Here's how the part is built. I have some questions about the finished solid (model axes, mm). Face numbers are marked on the shaded views. A direction names the side the tool comes from. Round coordinates to 2 decimals unless told otherwise and drop trailing zeros. Write each loop counter-clockwise with the first axis right and the second up, starting at its lowest first coordinate (ties: lowest second). Pieces come first, ordered by that corner, then holes. Notation, with made-up numbers: (55.5, -40) -> (100.5, -40) arc R25 cw to (100.5, -1) -> close; hole circle Ø5 at (-11.75, 45). An arc over 180 degrees is marked (long way). Put each result on its own line as item: value. Start each with the question number.
1) I want a section at C-C, the plane z = 10.25. List the corners of the cut face in (x, y) for me (3 decimals).
2) I want a section at D-D, the plane z = 4.75. List the corners of the cut face in (x, y) for me.
3) We'd pull the mould along X, two halves only. Please class the marked faces 3, 4, 5 and 6: released by +X, released by -X, zero draft, split by the parting line, or undercut.
4) If I drill on line 1 along Y through (x, z) = (0.25, 4.75); line 2 along Y through (x, z) = (0, 12.2) (3 decimals); line 3 along Z through (x, y) = (9.5, 2), over which ranges is the centre line in solid material (lowest first)? Write a range as [from, to].
5) Which directions (+Z, -Z, +X, -X, +Y, -Y) give clear straight access to the entire face, cutting with the end or side of a thin tool? Please do the marked faces 1 and 2.
6) Will these pins go through, and if not, where does the flat tip stop? P1, Ø1.5, axis at x = 1.5, z = 6.5, coming from the +Y side; P2, Ø10.5, axis at x = -1.5, y = 1, coming from the +Z side; P3, Ø3, axis at x = 7, z = 5.5, coming from the -Y side; P4, Ø1.5, axis at y = -5.5, z = 7, coming from the +X side.
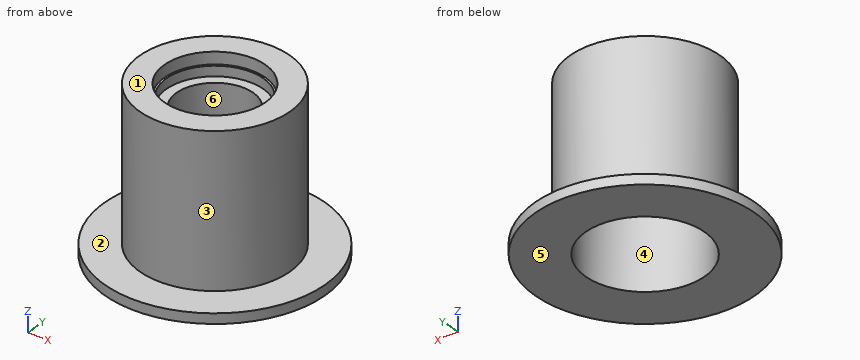
from build123d import *

# Parameters (mm, degrees)
F0_R         = 11
F1_DEPTH     = 1
F2_R         = 7.5
F3_DEPTH     = 15
F4_R         = 3.825
F5_DEPTH     = 25
F6_R         = 5.95
F7_DEPTH     = 7.3
F8_R         = 5.0375
F8_R_2       = 3.825
F9_DEPTH     = 1.2
F10_S5_R     = 5.95
F10_T6_DEPTH = 10
F11_R        = 4.834999796
F11_R_2      = 3.825
F12_DEPTH    = 1


# Not quite as in the source:
# - a fillet or chamfer that OpenCascade refuses, or shapes differently, is made with other operations: its cross-section is extruded or revolved along the edge and cut away or added


with BuildPart() as f1:
    # F0 (on Top) → F1 (new body)
    with BuildSketch(Plane.XY):
        Circle(F0_R)
    extrude(amount=F1_DEPTH)

    # F2 (on face) → F3 (join)
    with BuildSketch(Plane.XY.offset(1)):
        Circle(F2_R)
    extrude(amount=F3_DEPTH)

    # F4 (on face) → F5 (cut)
    with BuildSketch(Plane.XY.offset(16)):
        Circle(F4_R)
    extrude(amount=-F5_DEPTH, mode=Mode.SUBTRACT)

    # F6 (on face) → F7 (cut)
    with BuildSketch(Plane(origin=(0, 0, 0), x_dir=(1, 0, 0), z_dir=(0, 0, -1))):
        Circle(F6_R)
    extrude(amount=-F7_DEPTH, mode=Mode.SUBTRACT)

    # F8 (on face) → F9 (cut)
    with BuildSketch(Plane.XY.offset(16)):
        Circle(F8_R)
        Circle(F8_R_2, mode=Mode.SUBTRACT)
    extrude(amount=-F9_DEPTH, mode=Mode.SUBTRACT)

    # F10: chamfer of 2.2 x 2 on 1 edges, made by hand


with BuildPart() as f10_tool2:
    # F10_s3 → F10_t4 (revolve)
    with BuildSketch(Plane.XZ):
        Polygon((6.025, 7.3), (3.825, 9.3), (3.825, 7.3), align=None)
    revolve(axis=Axis((0, 0, 7.3), (0, 0, 1)))

    # F10_s5 → F10_t6 (intersect, symmetric)
    with BuildSketch(Plane.XY.offset(8.3)):
        Circle(F10_S5_R)
    extrude(amount=F10_T6_DEPTH, both=True, mode=Mode.INTERSECT)


with BuildPart() as f1_1:
    add(f1.part)

    # F10_t1: cut F10_tool2
    add(f10_tool2.part, mode=Mode.SUBTRACT)

    # F11 (on face) → F12 (cut)
    with BuildSketch(Plane.XY.offset(14.8)):
        Circle(F11_R)
        Circle(F11_R_2, mode=Mode.SUBTRACT)
    extrude(amount=-F12_DEPTH, mode=Mode.SUBTRACT)


solid = f1_1.part
Findings:
1. outline: circle Ø15 at (0, 0); hole circle Ø7.65 at (0, 0)
2. outline: circle Ø15 at (0, 0); hole circle Ø11.9 at (0, 0)
3. face 3: split by the parting line
3. face 4: undercut
3. face 5: zero draft
3. face 6: undercut
4. line 1: y = [-7.5, -5.94], [5.94, 7.5]
4. line 2: y = [-7.5, -3.825], [3.825, 7.5]
4. line 3: z = [0, 1]
5. face 1: +Z, +X, -X, +Y, -Y
5. face 2: +Z
6. P1: stops at y = 7.46
6. P2: stops at z = 16
6. P3: stops at y = -5.1
6. P4: stops at x = 5.8
